Part print with two shaded views. Sizes in mm from the minimum x, y, z corner. Give positions to 0.01 mm unless a question says otherwise; leave off trailing zeros. Loops run counter-clockwise (first coordinate to the right, second up) from the corner with the lowest first, then second, coordinate; pieces in that order, holes last. Notation, with made-up numbers: (-37, 52.5) -> (-27, 52.5) arc R28 cw to (-27, 89.5) -> close; hole circle Ø8 at (18, -9.5). An arc over 180 degrees is marked (long way). One line per question, with ' | ' between items. Start each with the question number.
(1) Slice it at D-D, the plane x = 14.75. Write the cut outline in (y, z), then the cut area to 3 significant figures.
(2) Slice it at B-B, the plane z = 1.15. Write the cut outline in (x, y).
(3) Slice it at A-A, the plane x = 8. Write the cut outline in (y, z), then the cut area to 3 significant figures.
(4) Slice it at C-C, the plane y = 14. Write the cut outline in (x, z), then the cut area to 3 significant figures.
(5) Drill centre lines: L1, parallel to X at y = 8.5, z = 0.1; L2, parallel to Y at x = 8.25, z = 1.4. Where is each one in solid material? Low to high. Write a range as from..to.
(6) Mould opens along Y. For the marked faces 1, 2 and 3 say: pulls with the +Y half, pulls with the -Y half, needs draft (parallel to the pull), parting line crosses it, or undercut.
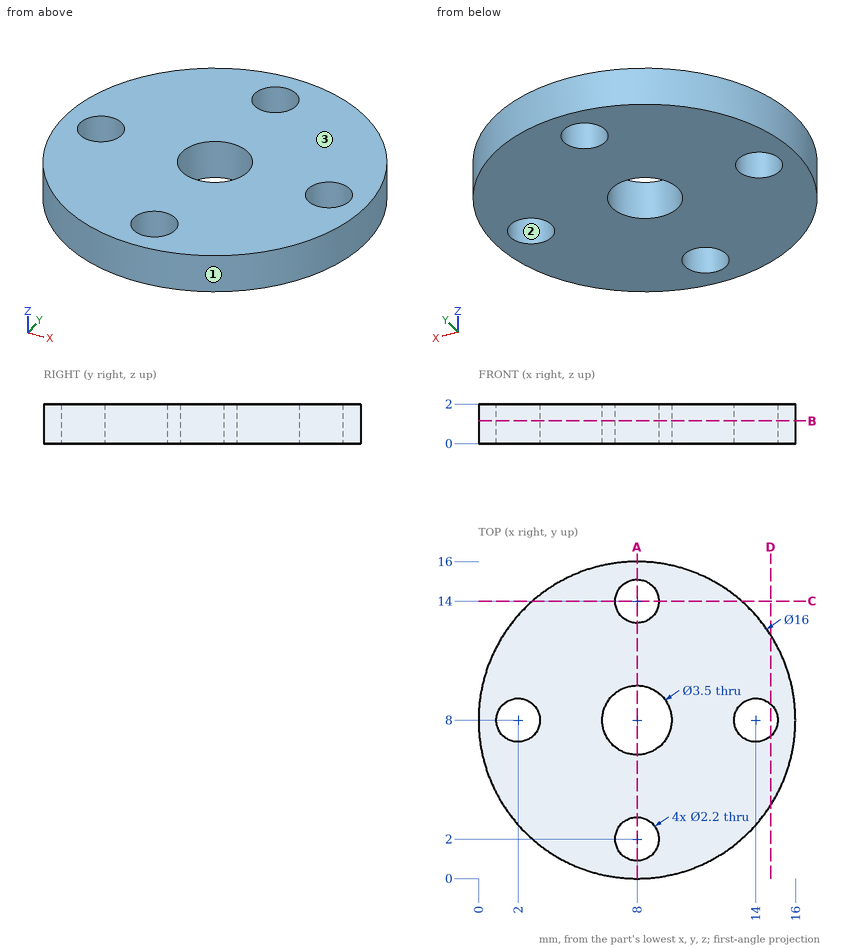
Final values:
1) outline: (3.71, 0) -> (7.2, 0) -> (7.2, 2) -> (3.71, 2) -> close; (8.8, 0) -> (12.29, 0) -> (12.29, 2) -> (8.8, 2) -> close | area: 14.0 mm2
2) outline: circle Ø16 at (8, 8); hole circle Ø2.2 at (2, 8); hole circle Ø3.5 at (8, 8); hole circle Ø2.2 at (8, 2); hole circle Ø2.2 at (8, 14); hole circle Ø2.2 at (14, 8)
3) outline: (0, 0) -> (0.9, 0) -> (0.9, 2) -> (0, 2) -> close; (3.1, 0) -> (6.25, 0) -> (6.25, 2) -> (3.1, 2) -> close; (9.75, 0) -> (12.9, 0) -> (12.9, 2) -> (9.75, 2) -> close; (15.1, 0) -> (16, 0) -> (16, 2) -> (15.1, 2) -> close | area: 16.2 mm2
4) outline: (2.71, 0) -> (6.9, 0) -> (6.9, 2) -> (2.71, 2) -> close; (9.1, 0) -> (13.29, 0) -> (13.29, 2) -> (9.1, 2) -> close | area: 16.8 mm2
5) L1: 0.02..1.02, 2.98..6.32, 9.68..13.02, 14.98..15.98 | L2: 0..0.93, 3.07..6.27, 9.73..12.93, 15.07..16
6) face 1: parting line crosses it | face 2: undercut | face 3: needs draft
